Check sheet for the modelled part. Datum: model origin and axes. Units: mm. Round coordinates to 2 decimals unless told otherwise and drop trailing zeros. Write each loop counter-clockwise with the first axis right and the second up, starting at its lowest first coordinate (ties: lowest second). Pieces come first, ordered by that corner, then holes.
Item 1: Depth check by flat-ended pin: pin 1 (1.5 mm diameter, centred on x = -2.5, y = 82.5, fed in from -Z); pin 2 (5 mm diameter, centred on x = -1.5, z = 1.5, fed in from -Y); pin 3 (1 mm diameter, centred on y = 120, z = 1, fed in from +X). Enter the tip coordinate at first touch or a pass-through.
Item 2: Material ranges on line 1 along Y through (x, z) = (2.5, -3.5); line 2 along Y through (x, z) = (1.5, -4.5); line 3 along X through (y, z) = (75.5, -0.25), recorded low to high.
Item 3: Section check A-A, the plane y = 117.5. Record the cut outline in (x, z).
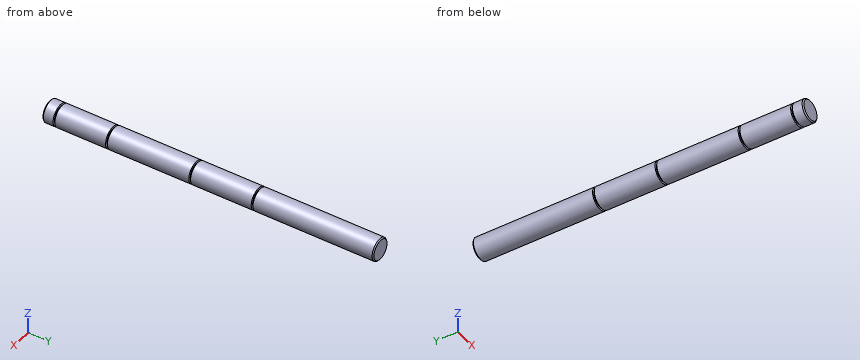
from build123d import *

# Parameters (mm, degrees)
SKETCH1_R           = 5
BOSS_EXTRUDE1_DEPTH = 150
CHAMFER1_SIZE       = 0.5
SKETCH2_W           = 1
SKETCH2_H           = 0.8
LPATTERN1_COUNT     = 2
LPATTERN1_PITCH     = 28.3
SKETCH3_W           = 1
SKETCH3_H           = 0.8


with BuildPart() as part:
    # Sketch1 → Boss-Extrude1 (new body)
    with BuildSketch(Plane(origin=(0, 0, 0), x_dir=(1, 0, 0), z_dir=(0, 1, 0))):
        with Locations(Location((0, 0, 0), (0, 0, 270))):
            Circle(SKETCH1_R)
    extrude(amount=BOSS_EXTRUDE1_DEPTH)

    # Chamfer1
    chamfer1_edges = [part.edges().sort_by_distance(p)[0] for p in [
        (0, 0, -5),
        (0, 150, -5),
    ]]
    chamfer(chamfer1_edges, length=CHAMFER1_SIZE)

    # Sketch2 → Cut-Revolve1 (revolve, cut)
    with BuildSketch(Plane.XY, mode=Mode.PRIVATE) as cut_revolve1_sk:
        with Locations((-4.5, 66.8)):
            Rectangle(SKETCH2_W, SKETCH2_H)
    cut_revolve1 = revolve(cut_revolve1_sk.sketch.rotate(Axis((0, 141.907824912, 0), (0, -1, 0)), 270), axis=Axis((0, 141.907824912, 0), (0, -1, 0)), mode=Mode.SUBTRACT)

    # LPattern1: Cut-Revolve1 ×2
    with Locations(*[(0, i * LPATTERN1_PITCH, 0) for i in range(1, LPATTERN1_COUNT)]):
        add(cut_revolve1, mode=Mode.SUBTRACT)

    # Sketch3 → Cut-Revolve2 (revolve, cut)
    with BuildSketch(Plane.XY, mode=Mode.PRIVATE) as cut_revolve2_sk:
        with Locations((-4.5, 5.3)):
            Rectangle(SKETCH3_W, SKETCH3_H)
        with Locations((-4.5, 29.1)):
            Rectangle(SKETCH3_W, SKETCH3_H)
    revolve(cut_revolve2_sk.sketch.rotate(Axis((0, 152.904561978, 0), (0, -1, 0)), 270), axis=Axis((0, 152.904561978, 0), (0, -1, 0)), mode=Mode.SUBTRACT)


solid = part.part
Values found:
1. pin 1: stops at z = -4.68
1. pin 2: stops at y = 0
1. pin 3: stops at x = 4.97
2. line 1: y = 0 to 4.9, 5.7 to 28.7, 29.5 to 66.4, 67.2 to 94.7, 95.5 to 150
2. line 2: y = 0.24 to 4.9, 5.7 to 28.7, 29.5 to 66.4, 67.2 to 94.7, 95.5 to 149.76
2. line 3: x = -4.99 to 4.99
3. outline: circle Ø10 at (0, 0)
